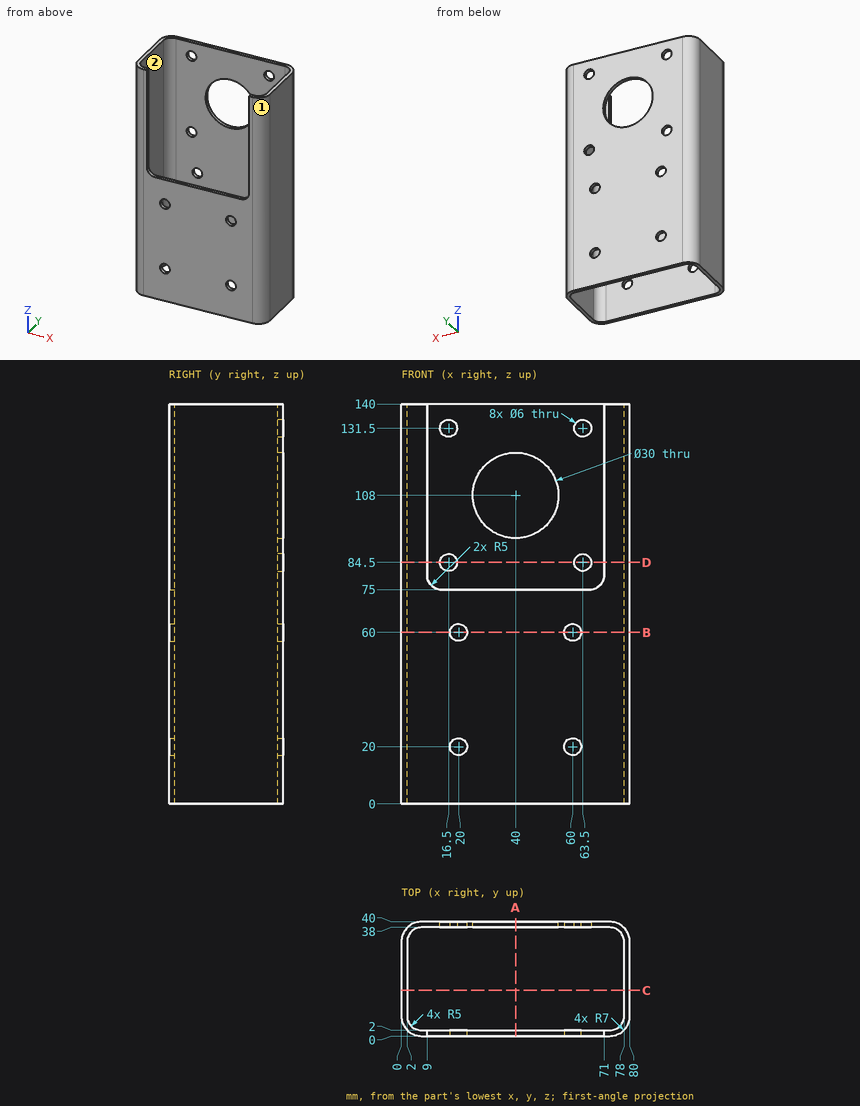
Study the drawing (mm; zero at the part's minimum x, y, z) and answer. A direction names the side the tool comes from. Round coordinates to 2 decimals unless told otherwise and drop trailing zeros. Write each loop counter-clockwise with the first axis right and the second up, starting at its lowest first coordinate (ties: lowest second). Pieces come first, ordered by that corner, then holes. Notation, with made-up numbers: (-8.5, -12.75) -> (-0.5, -12.75) arc R22 cw to (-0.5, -4.75) -> close; hole circle Ø10 at (-34, 67.5). An arc over 180 degrees is marked (long way). Write item = value, one per line.
1) Which of the six approach directions +Z, -Z, +X, -X, +Y, -Y give full straight-line access (tool end or side, diameter ignored) to the marked faces 1 and 2?
Check values:
face_1 = +Z, -Z, +X, -Y
face_2 = +Z, -Z
2) Section A-A on x = 40 is taken. Write down the section's boundary in (y, z).
Check values:
outline = (0, 0) -> (2, 0) -> (2, 75) -> (0, 75) -> close; (38, 0) -> (40, 0) -> (40, 93) -> (38, 93) -> close; (38, 123) -> (40, 123) -> (40, 140) -> (38, 140) -> close
3) Given pin 1 (9.5 mm diameter, centred on x = 60, z = 60, fed in from -Y); pin 2 (9.5 mm diameter, centred on x = 63.5, z = 84.5, fed in from -Y); pin 3 (2 mm diameter, centred on y = 1.5, z = 112, fed in from +X); pin 4 (0.6 mm diameter, centred on y = 1.5, z = 95, fed in from -X), each flat-ended and moving along its own axis, determine where each tip first touches the part or whether it passes through.
Check values:
pin_1 = 0
pin_2 = 38
pin_3 = 78.36
pin_4 = 2.31
4) Section B-B on z = 60 is taken. Give the number of separate pieces and of enclosed holes in the cut face, plus the area to 3 significant figures.
Check values:
separate_pieces = 4
enclosed_holes = 0
area = 395 mm²
5) Straight lines are drawn through the part: line 1 along Z through (x, y) = (20, 39.6); line 2 along Y through (x, z) = (47, 10); line 3 along X through (y, z) = (38.4, 84.5). For each, find the intervals that lie inside material, in ascending order. Write a range as [from, to].
Check values:
line_1 = [0, 17], [23, 57], [63, 140]
line_2 = [0, 2], [38, 40]
line_3 = [2.55, 13.5], [19.5, 60.5], [66.5, 77.45]
6) Section C-C on y = 16 is taken. Write down the section's boundary in (x, z).
Check values:
outline = (0, 0) -> (2, 0) -> (2, 140) -> (0, 140) -> close; (78, 0) -> (80, 0) -> (80, 140) -> (78, 140) -> close
7) Section D-D on z = 84.5 is taken. Write down the section's boundary in (x, y), plus the area to 3 significant figures.
Check values:
outline = (0, 7) arc R7 ccw to (7, 0) -> (9, 0) -> (9, 2) -> (7, 2) arc R5 cw to (2, 7) -> (2, 33) arc R5 cw to (7, 38) -> (13.5, 38) -> (13.5, 40) -> (7, 40) arc R7 ccw to (0, 33) -> close; (19.5, 38) -> (60.5, 38) -> (60.5, 40) -> (19.5, 40) -> close; (66.5, 38) -> (73, 38) arc R5 cw to (78, 33) -> (78, 7) arc R5 cw to (73, 2) -> (71, 2) -> (71, 0) -> (73, 0) arc R7 ccw to (80, 7) -> (80, 33) arc R7 ccw to (73, 40) -> (66.5, 40) -> close
area = 295 mm²
